from build123d import *

# Parameters (mm, degrees)
SKETCH1_R               = 3.175
BOSS_EXTRUDE1_DEPTH     = 41.91
CUT_EXTRUDE1_DEPTH      = 43.149844009
CUT_EXTRUDE1_DEPTH_BACK = 43.149844009
SKETCH2_R               = 1.905
CUT_EXTRUDE2_DEPTH      = 43.149844124
CUT_EXTRUDE2_DEPTH_BACK = 43.149844124
SKETCH3_R               = 1.905


with BuildPart() as part:
    # Sketch1 → Boss-Extrude1 (new body)
    with BuildSketch(Plane.XY):
        Circle(SKETCH1_R)
    extrude(amount=BOSS_EXTRUDE1_DEPTH)

    # Sketch2 → Cut-Extrude1 (cut, two sides: drawn at the far end of the back side and taken through both)
    with BuildSketch(Plane(origin=(0, 0, 0), x_dir=(1, 0, 0), z_dir=(0, 1, 0)).offset(-CUT_EXTRUDE1_DEPTH_BACK)):
        with Locations(Location((0, -32.639, 0), (0, 0, 270))):
            Circle(SKETCH2_R)
    extrude(amount=CUT_EXTRUDE1_DEPTH + CUT_EXTRUDE1_DEPTH_BACK, mode=Mode.SUBTRACT)

    # Sketch3 → Cut-Extrude2 (cut, two sides: drawn at the far end of the back side and taken through both)
    with BuildSketch(Plane(origin=(0, 0, 0), x_dir=(0, 0, -1), z_dir=(1, 0, 0)).offset(-CUT_EXTRUDE2_DEPTH_BACK)):
        with Locations((-4.303139223, 0)):
            Circle(SKETCH3_R)
    extrude(amount=CUT_EXTRUDE2_DEPTH + CUT_EXTRUDE2_DEPTH_BACK, mode=Mode.SUBTRACT)


solid = part.part
Can you work these out from the model? Positions are in its coordinate system, mm. Give positions to 0.01 mm unless a question says otherwise; leave off trailing zeros. Loops run counter-clockwise (first coordinate to the right, second up) from the corner with the lowest first, then second, coordinate; pieces in that order, holes last. Notation, with made-up numbers: (-17, 20) - (-3, 20) arc R19 ccw to (-3, 37) - close; hole circle Ø1 at (-21.75, -29). An arc over 180 degrees is marked (long way). Return JSON: item names as keys, results as strings.
1. I want a section at C-C on z = 7.5. Please give me the cut outline in (x, y) (3 decimals).
Output values:
{"outline": "circle Ø6.35 at (0, 0)"}
2. I want a section at A-A on x = 0. Please give me the cut outline in (y, z) (3 decimals), and give its area (3 significant figures).
Output values:
{"outline": "(-3.175, 0) - (3.175, 0) - (3.175, 30.734) - (-3.175, 30.734) - close; (-3.175, 34.544) - (3.175, 34.544) - (3.175, 41.91) - (-3.175, 41.91) - close; hole circle Ø3.81 at (0, 4.303)", "area": "231 mm²"}
3. I want a section at B-B on y = 0. Please give me the cut outline in (x, z) (3 decimals), and give its area (3 significant figures).
Output values:
{"outline": "(-3.175, 0) - (3.175, 0) - (3.175, 2.398) - (-3.175, 2.398) - close; (-3.175, 6.208) - (3.175, 6.208) - (3.175, 41.91) - (-3.175, 41.91) - close; hole circle Ø3.81 at (0, 32.639)", "area": "231 mm²"}
4. If I drill on line 1 (Z direction, x = 0, y = 1.5); line 2 (Z direction, x = -0.5, y = -0.25); line 3 (Z direction, x = 0, y = 2), over which ranges is the centre line in solid material (lowest first)?
Output values:
{"line 1": "z = 0 to 3.13, 5.48 to 30.73, 34.54 to 41.91", "line 2": "z = 0 to 2.41, 6.19 to 30.8, 34.48 to 41.91", "line 3": "z = 0 to 30.73, 34.54 to 41.91"}
5. We'd pull the mould along Z, two halves only. Please class faces 1 (the face through (-0.044, 0.084, 6.206)), 2 (the face through (0, 0, 0)), 3 (the face through (0, 0, 41.91)): +Z half, -Z half, draft (parallel to the pull), parting line (faces both ways), or undercut.
Output values:
{"face 1": "undercut", "face 2": "-Z half", "face 3": "+Z half"}
6. I want a section at D-D on x = -2.25. Please give me the cut outline in (y, z) (3 decimals).
Output values:
{"outline": "(-2.24, 0) - (2.24, 0) - (2.24, 41.91) - (-2.24, 41.91) - close; hole circle Ø3.81 at (0, 4.303)"}
